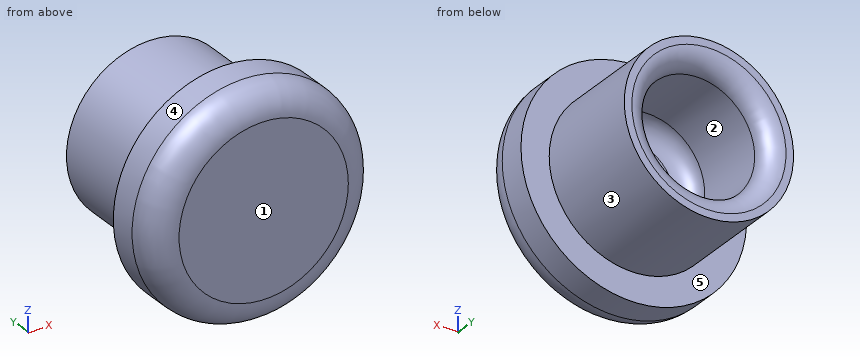
```python
from build123d import *

# Parameters (mm, degrees)
SKETCH_1_R        = 6
EXTRUDE_1_DEPTH   = 3
SKETCH_2_R        = 4.5
SKETCH_2_R_2      = 3.1
EXTRUDE_1_2_DEPTH = 6
FILLET_1_R        = 1
FILLET_2_R        = 1.5


with BuildPart() as part:
    # ｽｹｯﾁ1 → Extrude 1 (new body)
    with BuildSketch(Plane(origin=(0, 0, 0), x_dir=(1, 0, 0), z_dir=(0, 1, 0))):
        Circle(SKETCH_1_R)
    extrude(amount=EXTRUDE_1_DEPTH)

    # ｽｹｯﾁ2 → Extrude 1 2 (add)
    with BuildSketch(Plane(origin=(0, 3, 0), x_dir=(1, 0, 0), z_dir=(0, 1, 0))):
        Circle(SKETCH_2_R)
        Circle(SKETCH_2_R_2, mode=Mode.SUBTRACT)
    extrude(amount=EXTRUDE_1_2_DEPTH)

    # ﾌｨﾚｯﾄ1
    fillet_1_edges = [part.edges().sort_by_distance(p)[0] for p in [
        (-3.1, 3, 0),
        (-3.1, 9, 0),
    ]]
    fillet(fillet_1_edges, radius=FILLET_1_R)

    # ﾌｨﾚｯﾄ2
    fillet_2_edges = [part.edges().sort_by_distance(p)[0] for p in [
        (-6, 0, 0),
    ]]
    fillet(fillet_2_edges, radius=FILLET_2_R)


solid = part.part
```
For this review, take the finished solid that the model builds, in its own axes (mm). Face numbers are marked on the shaded views. A direction names the side the tool comes from. Round coordinates to 2 decimals unless told otherwise and drop trailing zeros. Write each loop counter-clockwise with the first axis right and the second up, starting at its lowest first coordinate (ties: lowest second). Pieces come first, ordered by that corner, then holes. Notation, with made-up numbers: (48.5, 8.25) - (68.5, 8.25) arc R16 cw to (68.5, 29.25) - close; hole circle Ø4 at (-17.5, 88.5). An arc over 180 degrees is marked (long way). Write each question's results on one line, items separated by ' | '.
Item 1: For pin 1 (3 mm diameter, centred on y = 6, z = -3.5, fed in from -X); pin 2 (3 mm diameter, centred on y = 2, z = -2.5, fed in from -X); pin 3 (1.5 mm diameter, centred on y = 7, z = 4, fed in from +X), all flat-tipped, find the tip position at first contact; note any pin that passes through.
Calculated:
pin 1: stops at x = -4.03 | pin 2: stops at x = -5.92 | pin 3: stops at x = 3.11
Item 2: Take a section at C-C on y = 5.5. State the section outline as (x, z) points, then the cut area to 3 significant figures.
Calculated:
outline: circle Ø9 at (0, 0); hole circle Ø6.2 at (0, 0) | area: 33.4 mm^2
Item 3: To check wall thickness, follow line 1 along X through (y, z) = (5.5, 0); line 2 along Y through (x, z) = (1, -4.5). State the ranges of each line that lie inside material, in increasing order. Write a range as from..to.
Calculated:
line 1: x = -4.5..-3.1, 3.1..4.5 | line 2: y = 0..3
Item 4: Take a section at B-B on z = 0. State the section outline as (x, y) points.
Calculated:
outline: (-6, 1.5) arc R1.5 ccw to (-4.5, 0) - (4.5, 0) arc R1.5 ccw to (6, 1.5) - (6, 3) - (4.5, 3) - (4.5, 9) - (4.1, 9) arc R1 ccw to (3.1, 8) - (3.1, 4) arc R1 cw to (2.1, 3) - (-2.1, 3) arc R1 cw to (-3.1, 4) - (-3.1, 8) arc R1 ccw to (-4.1, 9) - (-4.5, 9) - (-4.5, 3) - (-6, 3) - close
Item 5: For the marked faces 4 and 5, list the 3-axis set-ups (+Z, -Z, +X, -X, +Y, -Y) from which the entire face can be reached by the end or side of a thin tool; tool diameter is ignored.
Calculated:
face 4: +Y, -Y | face 5: +Y
Item 6: Take a section at D-D on y = 2. State the section outline as (x, z) points, then the cut area to 3 significant figures.
Calculated:
outline: circle Ø12 at (0, 0) | area: 113 mm^2
Item 7: Take a section at A-A on x = 0. State the section outline as (y, z) points.
Calculated:
outline: (0, -4.5) arc R1.5 ccw to (1.5, -6) - (3, -6) - (3, -4.5) - (9, -4.5) - (9, -4.1) arc R1 ccw to (8, -3.1) - (4, -3.1) arc R1 cw to (3, -2.1) - (3, 2.1) arc R1 cw to (4, 3.1) - (8, 3.1) arc R1 ccw to (9, 4.1) - (9, 4.5) - (3, 4.5) - (3, 6) - (1.5, 6) arc R1.5 ccw to (0, 4.5) - close
Item 8: Draft analysis for pull direction X (two halves, no side actions). For the marked faces 1, 2 and 3, state which applies: pulls with the +X half, pulls with the -X half, needs draft (parallel to the pull), parting line crosses it, or undercut.
Calculated:
face 1: needs draft | face 2: undercut | face 3: parting line crosses it
